Geometry: final body of the model. Coordinates: model frame, mm. A direction names the side the tool comes from. Round coordinates to 2 decimals unless told otherwise and drop trailing zeros. Order: outer loops, then holes, each group sorted by start corner. A loop starts at its lowest first (then second) coordinate and runs counter-clockwise, first axis right, second up. Notation, with made-up numbers: (-1, -15.5) - (56, -15.5) arc R17 ccw to (56, 10.5) - close; hole circle Ø2 at (-17, 60). An arc over 180 degrees is marked (long way). Put each result on its own line as item: value. Start each with the question number.
(1) Section B-B (z = -57). Output: boundary loops of the cut face in (x, y), and give its area (3 significant figures).
(2) Pull-direction query (Z, two-part tool) for faces 5 (the face through (-7, 9, -18)), 6 (the face through (-44, 17, -64)), 7 (the face through (-22, 16, -106)); classes: released by +Z, released by -Z, zero draft, split by the parting line, or undercut.
(3) Section D-D (x = -15.5). Output: boundary loops of the cut face in (y, z), and give its area (3 significant figures).
(4) Access query for faces 1 (the face through (-43, 29.5, -53)), 2 (the face through (-22, 4, 3)), 3 (the face through (-33, 1, -29)), 4 (the face through (-9, 2.5, -26)). Directions: +Z, -Z, +X, -X, +Y, -Y. A direction counts if a zero-diameter tool reaches every point of the face in a straight line with its end or side. Return the directions, or none.
(5) Pin query (flat end, axial travel): P1, Ø1, axis at x = -39, y = 17.5, coming from the -Z side; P2, Ø2, axis at y = 18.5, z = 3.5, coming from the +X side; P3, Ø1.1, axis at x = -21, y = 6, coming from the +Z side. Return the tip coordinate at first contact, or that it passes through.
(6) Section C-C (z = -32). Output: boundary loops of the cut face in (x, y).
(7) Material intervals for L1, parallel to Z at x = -43.1, y = 17.3; L2, parallel to Z at x = -8, y = 6; L3, parallel to X at y = 0.6, z = -5.5, sorted ascending. Write a range as [from, to].
(8) Section A-A (x = -6). Output: boundary loops of the cut face in (y, z).
Autodesk Inventor part; units mm, degrees
ref_plane "YZ Plane" through (0, 0, 0) normal (1, 0, 0) x (0, 1, 0)
ref_plane "XZ Plane" through (0, 0, 0) normal (0, 1, 0) x (-1, 0, 0)
ref_plane "XY Plane" through (0, 0, 0) normal (0, 0, 1) x (1, 0, 0)
sketch "внешние размеры" plane through (0, 0, 0) normal (0, 1, 0) x (-1, 0, 0)
  line L0 (0, 0) -> (44, 0)
  line L1 (44, 0) -> (44, -106)
  line L2 (44, -106) -> (0, -106)
  line L3 (0, -106) -> (0, 0)
  dimension "d0" = 44
  dimension "d1" = 106
extrude "Выдавливание1" add sketch "внешние размеры" along normal blind 33
sketch "внутренние размеры" plane through (0, 33, 0) normal (0, 1, 0) x (1, 0, 0)
  line L0 (-42, 2) -> (-2, 2)
  line L1 (-2, 2) -> (-2, 104)
  line L2 (-2, 104) -> (-42, 104)
  line L3 (-42, 104) -> (-42, 2)
  point P0 (0, 0)
extrude "Выдавливание2" cut sketch "внутренние размеры" against normal blind 30.5
sketch "перегородка" plane through (0, 2.5, 0) normal (0, 1, 0) x (1, 0, 0)
  line L0 (-42, 104) -> (-2, 104)
  line L1 (-20.5, 104) -> (-21.5, 104)
  line L2 (-21.5, 104) -> (-21.5, 54)
  line L3 (-21.5, 54) -> (-20.5, 54)
  line L4 (-20.5, 54) -> (-20.5, 104)
  line L5 (-2, 104) -> (-2, 2)
  line L6 (-42, 104) -> (-2, 104)
  point P0 (0, 0)
  point P1 (-22, 104)
  point P2 (-21, 54)
  dimension "d6" = 18.5
  dimension "d7" = 1
  dimension "d8" = 50
extrude "Выдавливание3" add sketch "перегородка" along normal blind 10
sketch "дисплей" plane through (-44, 0, -106) normal (-1, 0, 0) x (0, 0, 1)
  line L0 (45.5, 4) -> (59.5, 4)
  line L1 (59.5, 4) -> (59.5, 29.5)
  line L2 (59.5, 29.5) -> (45.5, 29.5)
  line L3 (45.5, 29.5) -> (45.5, 4)
  line L4 (0, 0) -> (0, 33)
  line L5 (0, 0) -> (106, 0)
  line L6 (0, 33) -> (106, 33)
  point P0 (0, 16.5)
  point P1 (59.5, 16.75)
  dimension "d21" = 25.5
  dimension "d22" = 14
  dimension "d23" = 45.5
  dimension "d24" = 4
  dimension "d25" = 3.5
  dimension "d125" = 59.5
extrude "Выдавливание4" cut sketch "дисплей" against normal blind 2.5
sketch "уф" plane through (-44, 0, -106) normal (-1, 0, 0) x (0, 0, 1)
  line L0 (80, 12.5) -> (72.5, 12.5)
  line L1 (72.5, 12.5) -> (72.5, 19)
  line L2 (72.5, 19) -> (80, 19)
  line L3 (80, 19) -> (80, 12.5)
  line L4 (106, 0) -> (106, 33)
  line L5 (0, 0) -> (106, 0)
  line L6 (0, 33) -> (106, 33)
  line L7 (0, 0) -> (0, 33)
  point P0 (80, 15.75)
  point P1 (72.5, 15.75)
  point P2 (0, 16.5)
  dimension "d28" = 7.5
  dimension "d29" = 6.5
  dimension "d30" = 26
  dimension "d31" = 12.5
  dimension "d32" = 14
  dimension "d126" = 72.5
extrude "Выдавливание5" cut sketch "уф" against normal blind 2.5 contours L0 L1 L2 L3
sketch "usb-c" plane through (0, 0, -106) normal (0, 0, -1) x (-1, 0, 0)
  line L0 (40.2, 24.8) -> (40.2, 15) construction
  line L1 (42, 4) -> (42, 29.5)
  line L2 (42, 23) -> (42, 16.8)
  line L3 (38.4, 16.8) -> (38.4, 23)
  arc A0 (42, 23) -> (38.4, 23) centre (40.2, 23) ccw
  arc A1 (38.4, 16.8) -> (42, 16.8) centre (40.2, 16.8) ccw
  line L4 (44, 0) -> (44, 33)
  line L5 (0, 0) -> (44, 0)
  point P0 (40.2, 19.9)
  point P1 (42, 19.9)
  point P2 (38.4, 19.9)
  point P3 (42, 16.8)
  point P4 (42, 23)
  dimension "d35" = 2
  dimension "d36" = 15
  dimension "d37" = 9.8
  dimension "d38" = 3.6
extrude "Выдавливание6" cut sketch "usb-c" against normal blind 2.5
sketch "stepper уши" plane through (0, 2.5, 0) normal (0, 1, 0) x (1, 0, 0)
  line L0 (-42, 2) -> (-42, 104)
  line L1 (-2, 2) -> (-42, 2)
  point P0 (0, 0)
  point P1 (-38.5, 5.5)
  point P2 (-15.5, 32)
  point P3 (-33, 24)
  point P4 (-33, 24)
  dimension "d41" = 3.5
  dimension "d42" = 3.5
  dimension "d43" = 26.5
  dimension "d44" = 30
  dimension "d45" = 35.0892
  dimension "d46" = 22
  dimension "d47" = 9
  dimension "d48" = 19.2419
  dimension "d49" = 19.3003
hole "Отверстие2" at (-33, 2.5, -24) at (-15.5, 2.5, -32) at (-38.5, 2.5, -5.5) at (-33, 2.5, -24) direction (0, -1, 0) diameter 2.5 depth 2.5 tip angle 118
sketch "stepper ось" plane through (0, 2.5, 0) normal (0, 1, 0) x (1, 0, 0)
  circle A0 centre (-33, 24) radius 1.25
  line L0 (-44, 0) -> (0, 0)
  line L1 (0, 0) -> (0, 106)
  dimension "d127" = 24
  dimension "d128" = 33
hole "Отверстие3" at (-33, 2.5, -24) direction (0, -1, 0) diameter 10 depth 2.5 tip angle 118
sketch "solar" plane through (0, 2.5, 0) normal (0, 1, 0) x (1, 0, 0)
  line L0 (-2, 104) -> (-2, 2)
  line L1 (-2, 2) -> (-8, 2)
  line L2 (-8, 2) -> (-8, 9.5)
  line L3 (-8, 9.5) -> (-2, 9.5)
  line L4 (-2, 9.5) -> (-2, 2)
  point P0 (0, 0)
  point P1 (-5, 2)
  point P2 (-5, 9.5)
  point P3 (-2, 9.5)
  dimension "d64" = 6
  dimension "d65" = 7.5
extrude "Выдавливание7" cut sketch "solar" against normal blind 2.5
sketch "кнопка" plane through (-44, 0, -106) normal (-1, 0, 0) x (0, 0, 1)
  line L0 (0, 0) -> (106, 0)
  line L1 (0, 0) -> (0, 33)
  point P0 (31.5, 17.3)
  dimension "d116" = 17.3
  dimension "d117" = 31.5
hole "Отверстие7" at (-44, 17.3, -74.5) direction (1, 0, 0) diameter 6.9 depth 2.5 tip angle 118
sketch "Эскиз25" plane through (-44, 0, -106) normal (-1, 0, 0) x (0, 0, 1)
  line L0 (106, 0) -> (106, 33)
  line L1 (106, 33) -> (110, 33)
  line L2 (110, 33) -> (110, 0)
  line L3 (110, 0) -> (106, 0)
  line L4 (106, 0) -> (106, 33)
extrude "Выдавливание12" add sketch "Эскиз25" against normal blind 44
sketch "паз" plane through (-44, 0, -106) normal (-1, 0, 0) x (0, 0, 1)
  line L0 (106, 33) -> (108, 33)
  line L1 (108, 33) -> (108, 2)
  line L2 (108, 2) -> (106, 2)
  line L3 (106, 2) -> (106, 33)
  line L4 (110, 33) -> (110, 0)
  line L5 (108, 33) -> (110, 33)
  line L6 (110, 33) -> (110, 4)
  line L7 (110, 4) -> (108, 4)
  line L8 (108, 4) -> (108, 33)
  point P0 (106, 0)
  point P1 (107, 2)
  point P2 (107, 33)
  point P3 (109, 4)
  point P4 (109, 33)
  dimension "d133" = 31
  dimension "d134" = 29
  dimension "d135" = 2
extrude "Выдавливание13" cut sketch "паз" against normal blind 44
sketch "Эскиз27" plane through (0, 2.5, 0) normal (0, 1, 0) x (1, 0, 0)
  line L0 (-42, 104) -> (-2, 104)
  line L1 (-18, 60) -> (-17, 60)
  line L2 (-17, 60) -> (-17, 104)
  line L3 (-17, 104) -> (-18, 104)
  line L4 (-18, 104) -> (-18, 60)
  point P0 (0, 0)
extrude "Выдавливание14" add sketch "Эскиз27" along normal blind 3 draft -10
sketch "Эскиз28" plane through (0, 2.5, 0) normal (0, 1, 0) x (1, 0, 0)
  line L0 (-2, 104) -> (-2, 2)
  line L1 (-2, 18) -> (-10, 18)
  line L2 (-10, 18) -> (-10, 19)
  line L3 (-10, 19) -> (-2, 19)
  line L4 (-2, 19) -> (-2, 18)
  line L5 (-2, 104) -> (-2, 9.5)
  line L6 (-2, 27) -> (-10, 27)
  line L7 (-10, 27) -> (-10, 28)
  line L8 (-10, 28) -> (-2, 28)
  line L9 (-2, 28) -> (-2, 27)
  line L10 (-10, 28) -> (-11, 28)
  line L11 (-11, 28) -> (-11, 18)
  line L12 (-11, 18) -> (-10, 18)
  line L13 (-10, 18) -> (-10, 28)
  point P0 (0, 0)
  point P1 (-2, 19)
extrude "Выдавливание15" add sketch "Эскиз28" along normal blind 13.5 contours L0 L6 L7 L8 | L7 L13 L2 L12 L11 L10 | L0 L1 L2 L3
sketch "кнопка2" plane through (0, 2.5, 0) normal (0, 1, 0) x (1, 0, 0)
  circle A0 centre (-6, 23) radius 3.6
  line L0 (0, -4) -> (0, 106)
  line L1 (-2, 19) -> (-10, 19)
  point P0 (0, 0)
  dimension "d147" = 7.2
  dimension "d172" = 6
  dimension "d173" = 4
hole "Отверстие9" at (-6, 2.5, -23) direction (0, -1, 0) diameter 7.2 depth 2.5 tip angle 118
sketch "Эскиз31" plane through (0, 2.5, 0) normal (0, 1, 0) x (1, 0, 0)
  line L0 (-2, 104) -> (-2, 2)
  line L1 (-2, 2) -> (-42, 2)
  line L2 (-2, 10) -> (-3, 10)
  line L3 (-3, 10) -> (-3, 2)
  line L4 (-3, 2) -> (-2, 2)
  line L5 (-2, 2) -> (-2, 10)
  point P0 (0, 0)
extrude "Выдавливание16" add sketch "Эскиз31" along normal blind 2
sketch "Эскиз32" plane through (-44, 4, 4) normal (0, 1, 0) x (1, 0, 0)
  line L0 (0, 0) -> (44, 0)
  line L1 (44, 4) -> (40, 4)
  line L2 (40, 0) -> (44, 0)
  line L3 (44, 0) -> (44, 4)
  line L4 (0, 110) -> (0, 0)
  line L5 (0, 4) -> (44, 4)
  line L6 (0, 0) -> (4, 0)
  line L7 (4, 0) -> (4, 4)
  line L8 (4, 4) -> (0, 4)
  line L9 (0, 4) -> (0, 0)
  point P0 (4, 0)
extrude "Выдавливание17" add sketch "Эскиз32" along normal blind 29 contours L4 L5 L7 L0
sketch "Эскиз33" plane through (0, 4, 4) normal (0, 1, 0) x (1, 0, 0)
  line L0 (0, 4) -> (-4, 4)
  line L1 (-4, 4) -> (-4, 0)
  line L2 (-4, 0) -> (0, 0)
  line L3 (0, 0) -> (0, 4)
extrude "Выдавливание18" add sketch "Эскиз33" along normal blind 12
sketch "Эскиз34" plane through (0, 16, 4) normal (0, 1, 0) x (1, 0, 0)
  line L0 (-44, 2) -> (0, 2)
  line L1 (-40, 4) -> (0, 4)
  line L2 (-1.6, 2) -> (-4, 2)
  line L3 (-4, 2) -> (-4, 4)
  line L4 (-4, 4) -> (-1.6, 4)
  line L5 (-1.6, 4) -> (-1.6, 2)
  line L6 (-40, 2) -> (-42, 2)
  line L7 (-42, 2) -> (-42, 4)
  line L8 (-42, 4) -> (-40, 4)
  line L9 (-40, 4) -> (-40, 2)
  point P0 (-1.6, 4)
  point P1 (-4, 2)
  point P2 (-1.6, 3)
  point P3 (-4, 3)
  point P4 (-2.8, 2)
  point P5 (-2.8, 4)
  dimension "d169" = 2.4
  dimension "d170" = 2
extrude "Выдавливание19" cut sketch "Эскиз34" against normal blind 15 contours L3 L1 L5 L0
sketch "Эскиз35" plane through (0, 33, 0) normal (0, 1, 0) x (1, 0, 0)
  line L0 (-40, -2) -> (-4, -2)
  line L1 (-40, 0) -> (-44, 0)
  line L2 (-40, -2) -> (-42, -2)
  line L3 (-42, -2) -> (-42, 0)
  line L4 (-42, 0) -> (-40, 0)
  line L5 (-40, 0) -> (-40, -2)
  point P0 (0, 0)
  point P1 (-40, -1)
  point P2 (-42, -1)
  dimension "d171" = 2
extrude "Выдавливание20" cut sketch "Эскиз35" against normal blind 31
sketch "Эскиз36" plane through (-44, 0, -106) normal (-1, 0, 0) x (0, 0, 1)
  line L0 (108, 33) -> (108, 4)
  line L1 (106, 2) -> (108, 2)
  line L2 (108, 4) -> (106, 4)
  line L3 (106, 4) -> (106, 2)
  line L4 (106, 2) -> (108, 2)
  line L5 (108, 2) -> (108, 4)
  point P0 (106, 0)
extrude "Выдавливание21" add sketch "Эскиз36" against normal blind 2
sketch "Эскиз37" plane through (0, 0, -106) normal (1, 0, 0) x (0, 0, -1)
  line L0 (-108, 2) -> (-108, 4)
  line L1 (-106, 4) -> (-106, 2)
  line L2 (-108, 4) -> (-106, 4)
  line L3 (-106, 4) -> (-106, 2)
  line L4 (-106, 2) -> (-108, 2)
  line L5 (-108, 2) -> (-108, 4)
  point P0 (-106, 0)
extrude "Выдавливание22" add sketch "Эскиз37" against normal blind 2
properties part number "roller_box_new03_10_2025"
Checks:
1. outline: (-44, 0) - (0, 0) - (0, 33) - (-2, 33) - (-2, 2.5) - (-20.5, 2.5) - (-20.5, 12.5) - (-21.5, 12.5) - (-21.5, 2.5) - (-42, 2.5) - (-42, 4) - (-44, 4) - close; (-44, 29.5) - (-42, 29.5) - (-42, 33) - (-44, 33) - close
1. area: 191 mm²
2. face 5: undercut
2. face 6: zero draft
2. face 7: released by -Z
3. outline: (0, -106) - (33, -106) - (33, -104) - (2.5, -104) - (2.5, -33.25) - (0, -33.25) - close; (0, -30.75) - (2.5, -30.75) - (2.5, -2) - (33, -2) - (33, 0) - (2, 0) - (2, 2) - (4, 2) - (4, 4) - (0, 4) - close
3. area: 393 mm²
4. face 1: -X
4. face 2: +Z, +Y
4. face 3: +Y, -Y
4. face 4: +Y
5. P1: stops at z = -2
5. P2: stops at x = -40
5. P3: stops at z = 0
6. outline: (-44, 0) - (-16.75, 0) - (-16.75, 2.5) - (-42, 2.5) - (-42, 12.5) - (-44, 12.5) - close; (-44, 19) - (-42, 19) - (-42, 33) - (-44, 33) - close; (-14.25, 0) - (0, 0) - (0, 33) - (-2, 33) - (-2, 2.5) - (-14.25, 2.5) - close
7. L1: z = [-106, -77.95], [-71.05, -60.5], [-46.5, -33.5], [-26, 4]
7. L2: z = [-106, -104], [-28, -27], [-19, -18], [-2, 0]
7. L3: x = [-44, -39.75], [-37.25, -8], [-2, 0]
8. outline: (0, -106) - (33, -106) - (33, -104) - (2.5, -104) - (2.5, -28) - (16, -28) - (16, -27) - (2.5, -27) - (2.5, -26.6) - (0, -26.6) - close; (0, -19.4) - (2.5, -19.4) - (2.5, -19) - (16, -19) - (16, -18) - (2.5, -18) - (2.5, -9.5) - (0, -9.5) - close; (0, -2) - (33, -2) - (33, 0) - (2, 0) - (2, 2) - (4, 2) - (4, 4) - (0, 4) - close
